Autodesk Inventor part; units mm, degrees
ref_plane "YZ Plane" through (0, 0, 0) normal (1, 0, 0) x (0, 1, 0)
ref_plane "XZ Plane" through (0, 0, 0) normal (0, 1, 0) x (-1, 0, 0)
ref_plane "XY Plane" through (0, 0, 0) normal (0, 0, 1) x (1, 0, 0)
sketch "스케치1" plane through (0, 0, 0) normal (0, 0, 1) x (1, 0, 0)
  circle A0 centre (0, 0) radius 38.5
  circle A1 centre (0, 0) radius 40
  dimension "d0" = 77
  dimension "d1" = 80
extrude "돌출1" add sketch "스케치1" along normal blind 20 contours A0 | A1
sketch "스케치2" plane through (0, 0, 0) normal (0, 0, -1) x (-1, 0, 0)
  circle A0 centre (0, 0) radius 38.5
  circle A1 centre (0, 0) radius 38.5
  dimension "d4" = 77
  dimension "d7" = 77
extrude "돌출2" cut sketch "스케치2" against normal blind 17
sketch "스케치3" plane through (0, 0, 0) normal (0, 0, 1) x (1, 0, 0)
  circle A0 centre (0, 0) radius 38.5
  circle A1 centre (0, 0) radius 47.5
  dimension "d8" = 95
  dimension "d9" = 77
extrude "돌출3" add sketch "스케치3" against normal blind 2
sketch "스케치4" plane through (0, 0, -2) normal (0, 0, -1) x (-1, 0, 0)
  line L0 (-25.3897, 5) -> (-51.6103, 5)
  line L1 (-51.6103, 5) -> (-51.6103, -5)
  line L2 (-51.6103, -5) -> (-25.3897, -5)
  line L3 (-25.3897, -5) -> (-25.3897, 5)
  circle A0 centre (0, 0) radius 38.5
  line L4 (-25.3897, 5) -> (-51.6103, -5) construction
  line L5 (-51.6103, 5) -> (-25.3897, -5) construction
  point P0 (-38.5, 0)
  dimension "d12" = 26.2206
  dimension "d13" = 10
extrude "돌출4" cut sketch "스케치4" against normal blind 19 contours L3 L2 A0 L0 | A0 L2 L1 L0 picked at (-29.7477, -0.557)
properties part number "라이다소켓"
Verification items for the finished model (mm, model axes). A direction names the side the tool comes from. Give positions to 0.01 mm unless a question says otherwise; leave off trailing zeros. Write each loop counter-clockwise with the first axis right and the second up, starting at its lowest first coordinate (ties: lowest second). Pieces come first, ordered by that corner, then holes. Notation, with made-up numbers: M 53,-32 L 72,-32 A4 cw 72,-28 Z; hole C -18.75,0.25 d6. An arc over 180 degrees is marked long. Put each result on its own line as item: value. Start each with the question number.
1. Section check A-A (y = 0). Record the cut outline in (x, z), and give its area (4 significant figures).
2. Draft check along Y on faces 1 (the face through (-47.457, 2.018, -0.986)), 2 (the face through (39, -5, 4)), 3 (the face through (-25, 32, 0)). Enter one of: +Y half, -Y half, draft (parallel to the pull), parting line (faces both ways), or undercut.
3. Go/stop test with flat-tipped pins: pin 1 Ø3 at (x, y) = (25, -1.5) entering from -Z; pin 2 Ø6 at (x, z) = (27, 6) entering from +Y; pin 3 Ø12 at (y, z) = (34, 10) entering from -X; pin 4 Ø7 at (x, z) = (44.5, 6) entering from +Y. Record where each tip stops, or that it passes through.
4. Section check C-C (y = 17.5). Record the cut outline in (x, z).
5. Set-up check for faces 4 (the face through (39, 5, 5)), 5 (the face through (-8.67, 39.05, 9.86)), 6 (the face through (-1, 1, 20)), 7 (the face through (1, 1, 17)), 8 (the face through (-39, 0, -2)): record each of +Z, -Z, +X, -X, +Y, -Y from which the full face is reachable in a straight line by a thin tool's end or side.
6. Scan lines: line 1 along Y through (x, z) = (0, 3.75); line 2 along Z through (x, y) = (15, 43.5); line 3 along Z through (x, y) = (2.5, 25.5). Record each from-to range of solid material in increasing order. Write a range as [from, to].
7. Section check D-D (z = 12). Record the cut outline in (x, y).
8. Section check B-B (x = 0). Record the cut outline in (y, z), and give its area (3 significant figures).
Answer list:
1. outline: M -47.5,-2 L -38.5,-2 L -38.5,17 L 40,17 L 40,20 L -40,20 L -40,0 L -47.5,0 Z
1. area: 283.5 mm2
2. face 1: parting line
2. face 2: undercut
2. face 3: draft
3. pin 1: z = 17
3. pin 2: y = 32
3. pin 3: x = -28.57
3. pin 4: through
4. outline: M -44.16,-2 L -34.29,-2 L -34.29,17 L 34.29,17 L 34.29,-2 L 44.16,-2 L 44.16,0 L 35.97,0 L 35.97,20 L -35.97,20 L -35.97,0 L -44.16,0 Z
5. face 4: -Z, +X
5. face 5: +Z
5. face 6: +Z, +X, -X, +Y, -Y
5. face 7: -Z
5. face 8: -Z, +X, -X, +Y, -Y
6. line 1: [-40, -38.5], [38.5, 40]
6. line 2: [-2, 0]
6. line 3: [17, 20]
7. outline: M 38.17,-5 A38.5 cw long 38.17,5 L 39.69,5 A40 ccw long 39.69,-5 Z
8. outline: M -47.5,-2 L -38.5,-2 L -38.5,17 L 38.5,17 L 38.5,-2 L 47.5,-2 L 47.5,0 L 40,0 L 40,20 L -40,20 L -40,0 L -47.5,0 Z
8. area: 327 mm2
